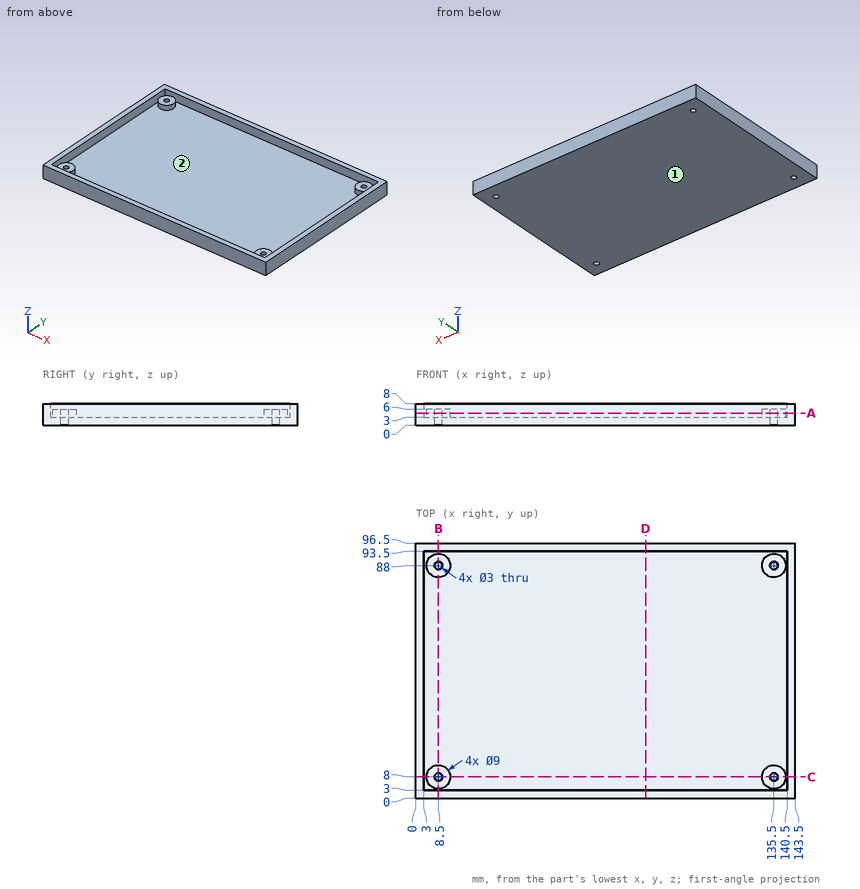
Job drawing, mm, ordinate dimensions from the low corner. One solid piece. Give positions to 0.01 mm unless a question says otherwise; leave off trailing zeros. Loops run counter-clockwise (first coordinate to the right, second up) from the corner with the lowest first, then second, coordinate; pieces in that order, holes last. Notation, with made-up numbers: (11, -7) -> (43, -7) arc R31 cw to (43, 29) -> close; hole circle Ø11 at (26.25, 87). An arc over 180 degrees is marked (long way). Use a Markdown table: item, result. Add a question column.
(1) Slice it at D-D on x = 87. List the corners of the cut face in (y, z).
(2) Slice it at C-C on y = 8. List the corners of the cut face in (x, z).
(3) Slice it at A-A on z = 4.5. Give the number of separate pieces and of enclosed holes in the cut face, and give its area (3 significant figures).
(4) Mould opens along Y. For the marked faces 1 and 2 say: +Y half, -Y half, draft (parallel to the pull), parting line (faces both ways), or undercut.
(5) Wall check: line 1 along Y through (x, z) = (8.5, 2.3); line 2 along X through (y, z) = (88, 2.1); line 3 along Y through (x, z) = (8.5, 3.6). Give the ranges that are in metal, low to high.
(6) Drop flat-ended pins along their axis: pin 1 Ø2 at (x, y) = (20.5, 54.5) entering from +Z; pin 2 Ø2.5 at (x, y) = (9, 6) entering from +Z. Give the stop position or say it passes through.
(7) Slice it at B-B on x = 8.5. List the corners of the cut face in (y, z).
Filled sheet:
| question | item | result |
|---|---|---|
| 1 | outline | (0, 0) -> (96.5, 0) -> (96.5, 8) -> (93.5, 8) -> (93.5, 3) -> (3, 3) -> (3, 8) -> (0, 8) -> close |
| 2 | outline | (0, 0) -> (7, 0) -> (7, 6) -> (4, 6) -> (4, 3) -> (3, 3) -> (3, 8) -> (0, 8) -> close; (10, 0) -> (134, 0) -> (134, 6) -> (131, 6) -> (131, 3) -> (13, 3) -> (13, 6) -> (10, 6) -> close; (137, 0) -> (143.5, 0) -> (143.5, 8) -> (140.5, 8) -> (140.5, 3) -> (140, 3) -> (140, 6) -> (137, 6) -> close |
| 3 | separate pieces | 5 |
| 3 | enclosed holes | 5 |
| 3 | area | 1,630 mm2 |
| 4 | face 1 | draft |
| 4 | face 2 | undercut |
| 5 | line 1 | 0 to 6.5, 9.5 to 86.5, 89.5 to 96.5 |
| 5 | line 2 | 0 to 7, 10 to 134, 137 to 143.5 |
| 5 | line 3 | 0 to 3, 3.5 to 6.5, 9.5 to 12.5, 83.5 to 86.5, 89.5 to 92.5, 93.5 to 96.5 |
| 6 | pin 1 | z = 3 |
| 6 | pin 2 | z = 6 |
| 7 | outline | (0, 0) -> (6.5, 0) -> (6.5, 6) -> (3.5, 6) -> (3.5, 3) -> (3, 3) -> (3, 8) -> (0, 8) -> close; (9.5, 0) -> (86.5, 0) -> (86.5, 6) -> (83.5, 6) -> (83.5, 3) -> (12.5, 3) -> (12.5, 6) -> (9.5, 6) -> close; (89.5, 0) -> (96.5, 0) -> (96.5, 8) -> (93.5, 8) -> (93.5, 3) -> (92.5, 3) -> (92.5, 6) -> (89.5, 6) -> close |
